CAD build for the part. Positions are in the model's coordinates, mm. A direction names the side the tool comes from. Round coordinates to 2 decimals unless told otherwise and drop trailing zeros. Order: outer loops, then holes, each group sorted by start corner. A loop starts at its lowest first (then second) coordinate and runs counter-clockwise, first axis right, second up. Notation, with made-up numbers: (70.25, 38) - (104.25, 38) arc R32 ccw to (104.25, 72) - close; hole circle Ø1 at (34, -6.5). An arc over 180 degrees is marked (long way). Write item = value, one per line.
from build123d import *

# Parameters (mm, degrees)
F0_R     = 9.525
F1_DEPTH = 25.4
F3_DEPTH = 3.175
F4_R     = 3.175
F5_DEPTH = 25.4


with BuildPart() as f1:
    # F0 (on Front) → F1 (new body)
    with BuildSketch(Plane.XZ):
        Polygon((-25.4, -12.7), (-25.4, 19.05), (-50.8, 19.05), (-50.8, -19.05), (50.8, -19.05), (50.8, -12.7), align=None)
        with Locations((-38.1, 6.35)):
            Circle(F0_R, mode=Mode.SUBTRACT)
    extrude(amount=F1_DEPTH)

    # F2 (on Front) → F3 (join)
    with BuildSketch(Plane.XZ):
        Polygon((50.8, -6.35), (-25.4, 19.05), (-25.4, -12.7), (50.8, -12.7), align=None)
    extrude(amount=F3_DEPTH)

    # F4 (on face) → F5 (cut)
    with BuildSketch(Plane.XY.offset(-12.7)):
        with Locations((39.6875, -14.2875)):
            Circle(F4_R)
        with Locations((-11.1125, -14.3002)):
            Circle(F4_R)
    extrude(amount=-F5_DEPTH, mode=Mode.SUBTRACT)

    # F6: F1 across plane


with BuildPart() as f1_1:
    add(f1.part)
    add(f1.part.mirror(Plane.XZ))


solid = f1_1.part
(1) Drop flat-ended pins along their axis: pin 1 (5.5 mm diameter, centred on x = -11.11, y = -14.3, fed in from +Z) (3 decimals); pin 2 (8.5 mm diameter, centred on x = -11.11, y = 14.3, fed in from +Z); pin 3 (9.5 mm diameter, centred on x = -0.5, z = -1.5, fed in from -Y) (3 decimals); pin 4 (1.5 mm diameter, centred on y = 14.5, z = -4.5, fed in from +X). Give the stop position or say it passes through.
Solved:
pin_1 = through
pin_2 = -12.7
pin_3 = -3.175
pin_4 = -25.4
(2) Band-saw the part on A-A on x = -38.1. List the corners of the cut face in (y, z) (3 decimals), plus the area to 3 significant figures.
Solved:
outline = (-25.4, -19.05) - (25.4, -19.05) - (25.4, -3.175) - (-25.4, -3.175) - close; (-25.4, 15.875) - (25.4, 15.875) - (25.4, 19.05) - (-25.4, 19.05) - close
area = 968 mm²
(3) Probe line 1 along Z through (x, y) = (-38.1, 10.5) (3 decimals); line 2 along X through (y, z) = (-15, -12); line 3 along Z through (x, y) = (45, -9). List the from-to ranges inside material, lowest first.
Solved:
line_1 = -19.05 to -3.175, 15.875 to 19.05
line_2 = -50.8 to -25.4
line_3 = -19.05 to -12.7
(4) Tool access for faces 1 (the flat face through (4, 3.175, 0)), 2 (the flat face through (4, -3.175, 0)), 3 (the flat face through (-27, -25.4, -8)): list every direction of +Z, -Z, +X, -X, +Y, -Y with a clear straight run to the whole face (end or side of a thin tool).
Solved:
face_1 = +Z, +X, +Y
face_2 = +Z, +X, -Y
face_3 = +Z, -Z, +X, -X, -Y
(5) Band-saw the part on D-D on x = 14.5. List the corners of the cut face in (y, z) (3 decimals), plus the area to 3 significant figures.
Solved:
outline = (-25.4, -19.05) - (25.4, -19.05) - (25.4, -12.7) - (3.175, -12.7) - (3.175, 5.75) - (-3.175, 5.75) - (-3.175, -12.7) - (-25.4, -12.7) - close
area = 440 mm²
(6) Band-saw the part on C-C on z = 9.5. List the corners of the cut face in (x, y) (3 decimals).
Solved:
outline = (-50.8, -25.4) - (-47.089, -25.4) - (-47.089, 25.4) - (-50.8, 25.4) - close; (-29.111, -25.4) - (-25.4, -25.4) - (-25.4, -3.175) - (3.25, -3.175) - (3.25, 3.175) - (-25.4, 3.175) - (-25.4, 25.4) - (-29.111, 25.4) - close
(7) Band-saw the part on B-B on y = 21. List the corners of the cut face in (x, z) (3 decimals), plus the area to 3 significant figures.
Solved:
outline = (-50.8, -19.05) - (50.8, -19.05) - (50.8, -12.7) - (-25.4, -12.7) - (-25.4, 19.05) - (-50.8, 19.05) - close; hole circle Ø19.05 at (-38.1, 6.35)
area = 1,170 mm²
(8) Pull direction X, two halves, no side cores. Call faces 4 (the cylindrical face through (41.394, 11.61, -15.831)), 5 (the cylindrical face through (-11.526, -11.152, -15.831)), 6 (the flat face through (13.233, -0.044, 6.172)), 7 (the flat face through (-38, 0, 19.05)): released by +X, released by -X, zero draft, split by the parting line, or undercut.
Solved:
face_4 = undercut
face_5 = undercut
face_6 = released by +X
face_7 = zero draft
